Could you check a few things on this model? Use its own coordinates, in mm. A direction names the side the tool comes from. Give positions to 0.01 mm unless a question says otherwise; leave off trailing zeros. Order: outer loops, then holes, each group sorted by start corner. A loop starts at its lowest first (then second) coordinate and runs counter-clockwise, first axis right, second up. Notation, with made-up numbers: M 65,63 L 112,63 A16 cw 112,75 Z; hole C 81.25,-38 d2. An arc over 180 degrees is marked long. Use a Markdown table: item, result. Add a question column.
Item 1: For faces 1 (the face through (4.525, -3.128, 0.014)), 2 (the face through (0.1, -20.615, 0.014)), 3 (the face through (5, -0.5, 0)), which set-ups out of +Z, -Z, +X, -X, +Y, -Y let a thin tool reach every point of the face, with its end or its side?
Item 2: If we mould it in two halves opening along Y, with no side actions, what happens to faces 4 (the face through (-2.889, -24.445, 0.014)), 5 (the face through (1.617, -0.67, -0.014)), 6 (the face through (-5, -11, 1))? For each: released by +Y, released by -Y, zero draft, split by the parting line, or undercut.
Item 3: Suppose I cut it at A-A on y = -19.75. Write out the boundary of the cut face in (x, z), plus the area to 3 significant figures.
Item 4: Suppose I cut it at C-C on x = 0. Write out the boundary of the cut face in (y, z), plus the area to 3 significant figures.
Item 5: Suppose I cut it at D-D on x = 3.75. Write out the boundary of the cut face in (y, z).
Item 6: I'm going to push flat-ended pins straight in: pin 1 Ø1 at (y, z) = (-10, 0.5) entering from -X; pin 2 Ø5.5 at (x, y) = (0, 0) entering from +Z; pin 3 Ø0.8 at (y, z) = (-0.5, 0) entering from +X; pin 4 Ø1.2 at (x, y) = (-4.94, -8.47) entering from -Z. Where does each tip first touch, or does it pass through?
Item 7: Suppose I cut it at B-B on z = 0.15. Write out the boundary of the cut face in (x, y), plus the area to 3 significant figures.
Item 8: If I drill on L1, parallel to Y at x = 0, z = 0.3; L2, parallel to Y at x = 2, z = -0.7; L3, parallel to Y at x = 3.75, z = -0.4, over which ranges is the centre line in solid material (lowest first)? Write a range as from..to.
from build123d import *

# Parameters (mm, degrees)
SKETCH1_R           = 1.75
SKETCH1_R_2         = 1
BOSS_EXTRUDE1_DEPTH = 1


with BuildPart() as part:
    # Sketch1 → Boss-Extrude1 (new, symmetric)
    with BuildSketch(Plane.XY):
        with BuildLine():
            Line((-5, 0), (-5, -2.928879346))
            ThreePointArc((-5, -2.928879346), (-5.462566041, -5.029282419), (-6.764677227, -6.741055438))
            Line((-6.764677227, -6.741055438), (-13.802331482, -12.713781389))
            ThreePointArc((-13.802331482, -12.713781389), (-15.555651524, -16.862770292), (-13.260540242, -20.738425628))
            ThreePointArc((-13.260540242, -20.738425628), (-2.732373515, -24.463408593), (8.3581995, -23.153071635))
            ThreePointArc((8.3581995, -23.153071635), (9.560275853, -20.592795782), (7, -19.39071943))
            ThreePointArc((7, -19.39071943), (0, -20.615528128), (-7, -19.39071943))
            ThreePointArc((-7, -19.39071943), (-8.933606572, -17.102043774), (-7.922544038, -14.28164962))
            Line((-7.922544038, -14.28164962), (3.235322773, -4.812176092))
            ThreePointArc((3.235322773, -4.812176092), (4.537433959, -3.100403073), (5, -1))
            Line((5, -1), (5, 0))
            ThreePointArc((5, 0), (0, 5), (-5, 0))
        make_face()
        Circle(SKETCH1_R, mode=Mode.SUBTRACT)
        with Locations((-4.935698975, -8.467802799)):
            Circle(SKETCH1_R_2, mode=Mode.SUBTRACT)
    extrude(amount=BOSS_EXTRUDE1_DEPTH, both=True)


solid = part.part
Findings below:
| question | item | result |
|---|---|---|
| 1 | face 1 | +Z, -Z, +X |
| 1 | face 2 | +Z, -Z |
| 1 | face 3 | +Z, -Z, +X, +Y |
| 2 | face 4 | released by -Y |
| 2 | face 5 | undercut |
| 2 | face 6 | zero draft |
| 3 | outline | M -14.39,-1 L -5.91,-1 L -5.91,1 L -14.39,1 Z; M 5.91,-1 L 8.98,-1 L 8.98,1 L 5.91,1 Z |
| 3 | area | 23.1 mm^2 |
| 4 | outline | M -24.62,-1 L -20.62,-1 L -20.62,1 L -24.62,1 Z; M -7.56,-1 L -1.75,-1 L -1.75,1 L -7.56,1 Z; M 1.75,-1 L 5,-1 L 5,1 L 1.75,1 Z |
| 4 | area | 26.1 mm^2 |
| 5 | outline | M -24.33,-1 L -20.27,-1 L -20.27,1 L -24.33,1 Z; M -4.31,-1 L 3.31,-1 L 3.31,1 L -4.31,1 Z |
| 6 | pin 1 | stops at x = -11.19 |
| 6 | pin 2 | stops at z = 1 |
| 6 | pin 3 | stops at x = 5 |
| 6 | pin 4 | passes through |
| 7 | outline | M -13.8,-12.71 A5 ccw -13.26,-20.74 A24.62 ccw 8.36,-23.15 A2 ccw 7,-19.39 A20.62 cw -7,-19.39 A3 cw -7.92,-14.28 L 3.24,-4.81 A5 ccw 5,-1 L 5,0 A5 ccw -5,0 L -5,-2.93 A5 cw -6.76,-6.74 Z; hole C -4.94,-8.47 d2; hole C 0,0 d3.5 |
| 7 | area | 267 mm^2 |
| 8 | L1 | y = -24.62..-20.62, -7.56..-1.75, 1.75..5 |
| 8 | L2 | y = -24.53..-20.52, -5.86..4.58 |
| 8 | L3 | y = -24.33..-20.27, -4.31..3.31 |
